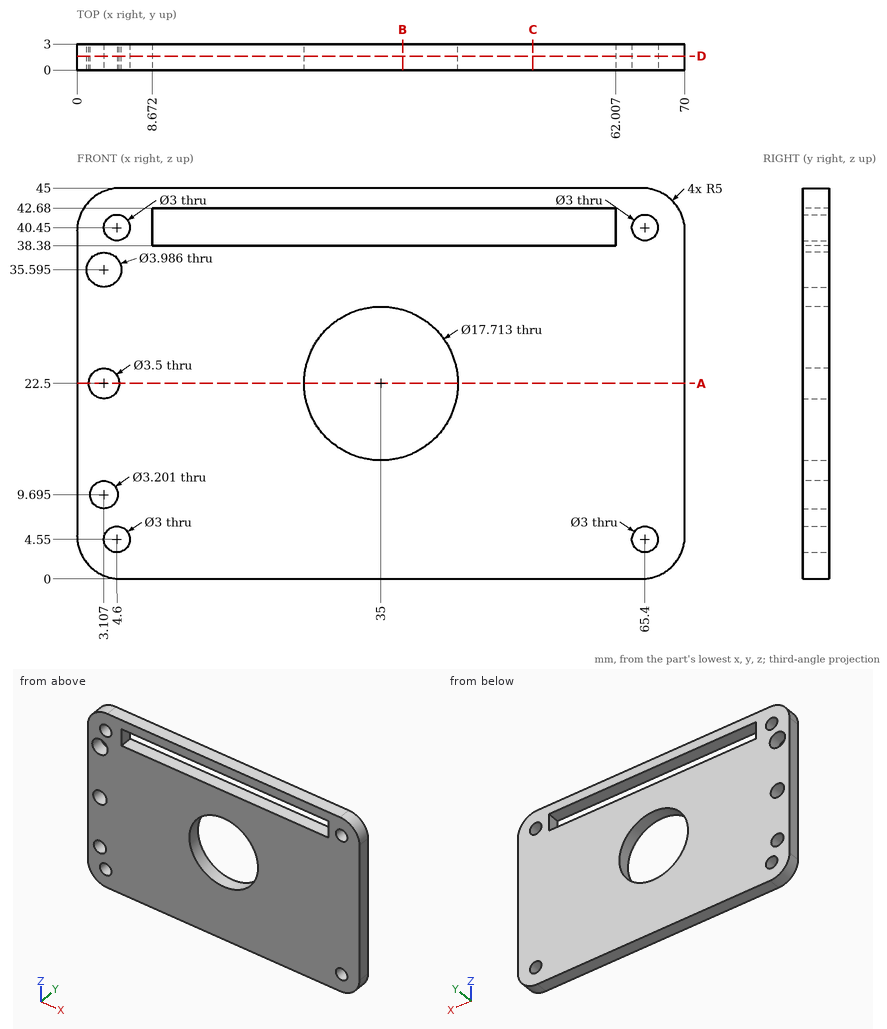
Here's the drawing with two shaded views (mm, measured from the low corner). I have some questions. Round coordinates to 2 decimals unless told otherwise and drop trailing zeros. Order: outer loops, then holes, each group sorted by start corner. A loop starts at its lowest first (then second) coordinate and runs counter-clockwise, first axis right, second up. Notation, with made-up numbers: M -6.5,88 L 33.5,88 A24 cw 33.5,120 Z; hole C 25,-39 d3. An arc over 180 degrees is marked long. Use CSV: the item, a comma, the result in double quotes.
1) I want a section at D-D (y = 1.6). Count the separate pieces of the cut face and the enclosed holes in it, then the cut area to 3 significant figures.
Taken from the geometry:
separate pieces,"1"
enclosed holes,"9"
area,"2,590 mm^2"
2) I need wall thicknesses on line 1 along Z through (x, y) = (65.5, 2) (1 decimal); line 2 along X through (y, z) = (1.8, 22.5); line 3 along X through (y, z) = (1.45, 40.45). Which ranges of each line are inside material? Lowest first, please. Write a range as [from, to].
Taken from the geometry:
line 1,"[0, 3.1], [6, 39], [41.9, 45]"
line 2,"[0, 1.36], [4.86, 26.14], [43.86, 70]"
line 3,"[0.02, 3.1], [6.1, 8.67], [62.01, 63.9], [66.9, 69.98]"
3) I want a section at A-A (z = 22.5). List the corners of the cut face in (x, y) for me.
Taken from the geometry:
outline,"M 0,0 L 1.36,0 L 1.36,3 L 0,3 Z; M 4.86,0 L 26.14,0 L 26.14,3 L 4.86,3 Z; M 43.86,0 L 70,0 L 70,3 L 43.86,3 Z"
4) I'm going to push flat-ended pins straight in: P1, Ø4, axis at x = 3.11, z = 9.69, coming from the +Y side; P2, Ø1.8, axis at x = 4.6, z = 4.55, coming from the +Y side. Where does each tip first touch, or does it pass through?
Taken from the geometry:
P1,"y = 3"
P2,"through"
5) I want a section at C-C (x = 52.5). List the corners of the cut face in (y, z) for me.
Taken from the geometry:
outline,"M 0,0 L 3,0 L 3,38.38 L 0,38.38 Z; M 0,42.68 L 3,42.68 L 3,45 L 0,45 Z"
6) I want a section at B-B (x = 37.5). List the corners of the cut face in (y, z) for me.
Taken from the geometry:
outline,"M 0,0 L 3,0 L 3,14 L 0,14 Z; M 0,31 L 3,31 L 3,38.38 L 0,38.38 Z; M 0,42.68 L 3,42.68 L 3,45 L 0,45 Z"
